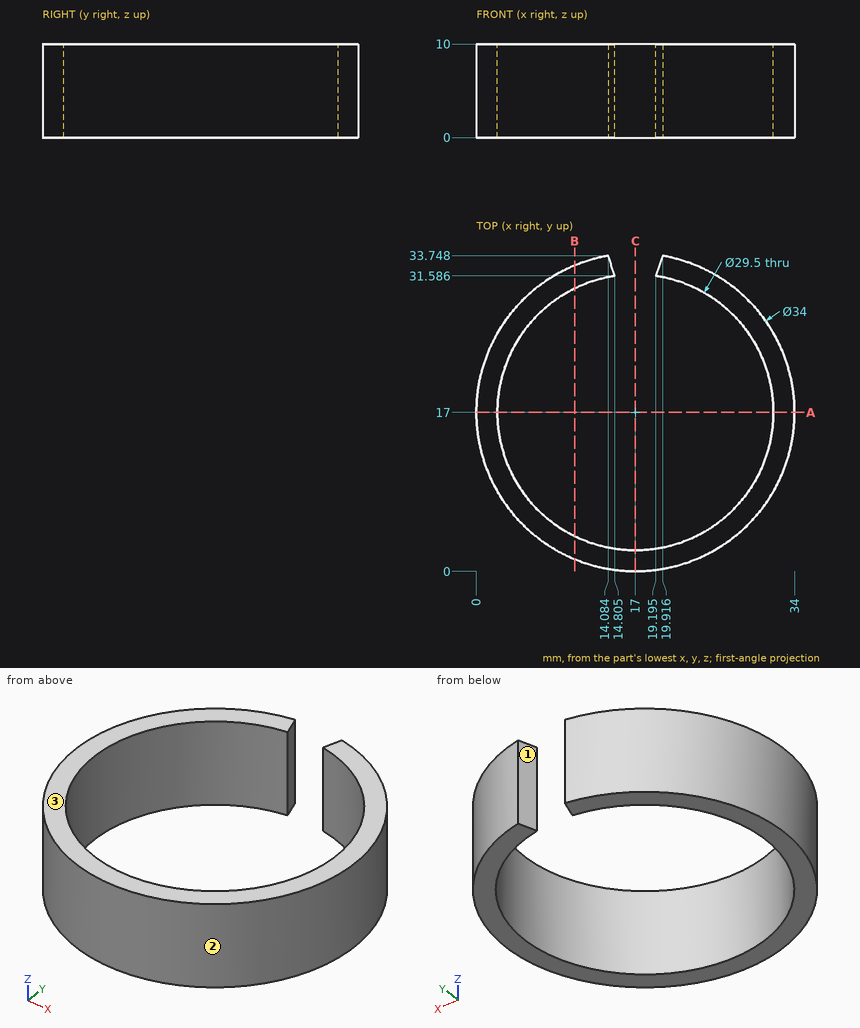
Answer from the drawing. Dimensions are ordinates in mm from the lowest x, y and z of the part. Coordinates: 2 decimals unless noted, no trailing zeros. Write each loop counter-clockwise with the first axis right and the second up, starting at its lowest first coordinate (ties: lowest second). Pieces come first, ordered by that corner, then holes. Notation, with made-up numbers: M 87,30.5 L 101,30.5 A20 cw 101,53.5 Z; hole C -18.5,35 d10. An arc over 180 degrees is marked long. Put each result on its own line as item: value. Start each with the question number.
1. For a pull along X with two mould halves and no side action, classify the marked faces 1, 2 and 3 as pulls with the +X half, pulls with the -X half, needs draft (parallel to the pull), parting line crosses it, or undercut.
2. A cutting plane is placed at B-B on x = 10.5. Write down the section's boundary in (y, z).
3. Consider line 1 (X direction, y = 17, z = 7.75); line 2 (X direction, y = 21, z = 9); line 3 (Y direction, x = 29, z = 1.5) (1 decimal). Determine where each line is inside the solid, lowest interval first. Write a range as from..to.
4. Flat-ended cylindrical pins translate along their axes: P1, Ø1.5, axis at y = 19.5, z = 3.5, coming from the -X side; P2, Ø4, axis at x = 12, z = 6, coming from the -Y side; P3, Ø1, axis at x = 22, z = 2, coming from the -Y side. Find the tip coordinate at first contact, or state that the pin passes through.
5. A cutting plane is placed at A-A on y = 17. Write down the section's boundary in (x, z), then the cut area to 3 significant figures.
6. A cutting plane is placed at C-C on x = 17. Write down the section's boundary in (y, z).
Resolved:
1. face 1: undercut
1. face 2: parting line crosses it
1. face 3: needs draft
2. outline: M 1.29,0 L 3.76,0 L 3.76,10 L 1.29,10 Z; M 30.24,0 L 32.71,0 L 32.71,10 L 30.24,10 Z
3. line 1: x = 0..2.25, 31.75..34
3. line 2: x = 0.48..2.8, 31.2..33.52
3. line 3: y = 5..8.4, 25.6..29
4. P1: stops at x = 0.09
4. P2: stops at y = 0.27
4. P3: stops at y = 0.61
5. outline: M 0,0 L 2.25,0 L 2.25,10 L 0,10 Z; M 31.75,0 L 34,0 L 34,10 L 31.75,10 Z
5. area: 45.0 mm2
6. outline: M 0,0 L 2.25,0 L 2.25,10 L 0,10 Z
